The listing builds one solid part. Answer for the finished solid, in the listing's coordinates (mm). Give positions to 0.01 mm unless a question says otherwise; leave off trailing zeros. Order: outer loops, then holes, each group sorted by start corner. A loop starts at its lowest first (then second) coordinate and runs counter-clockwise, first axis right, second up.
```python
from build123d import *

# Parameters (mm, degrees)
SKETCH1_R           = 9
SKETCH1_R_2         = 2.45
SKETCH1_R_3         = 1.5
BOSS_EXTRUDE1_DEPTH = 3


with BuildPart() as part:
    # Sketch1 → Boss-Extrude1 (new body)
    with BuildSketch(Plane(origin=(0, 0, 0), x_dir=(1, 0, 0), z_dir=(0, 1, 0))):
        Circle(SKETCH1_R)
        with Locations((-5, 0.000835232)):
            Circle(SKETCH1_R_2, mode=Mode.SUBTRACT)
        with Locations((2.999131959, -5.19665349)):
            Circle(SKETCH1_R_3, mode=Mode.SUBTRACT)
        with Locations((3.000867957, 5.195651211)):
            Circle(SKETCH1_R_3, mode=Mode.SUBTRACT)
        with BuildLine():
            Line((-1.499778997, 1.323126207), (-1.500220961, -1.322625067))
            ThreePointArc((-1.500220961, -1.322625067), (1.999999972, -0.000334093), (-1.499778997, 1.323126207))
        make_face(mode=Mode.SUBTRACT)
    extrude(amount=BOSS_EXTRUDE1_DEPTH)


solid = part.part
```
1) For a pull along Z with two mould halves and no side action, classify faces 1 (the flat face through (2, 3, 2)), 2 (the cylindrical face through (2.68, 1.48, -3.73)), 3 (the cylindrical face through (-1.172, 1.479, -8.923)) as +Z half, -Z half, draft (parallel to the pull), parting line (faces both ways), or undercut.
Geometry says:
face 1: draft
face 2: undercut
face 3: parting line
2) Find section C-C (x = 2.75). Write down the section's boundary in (y, z).
Geometry says:
outline: (0, -8.57) - (3, -8.57) - (3, -6.67) - (0, -6.67) - close; (0, -3.72) - (3, -3.72) - (3, 3.72) - (0, 3.72) - close; (0, 6.68) - (3, 6.68) - (3, 8.57) - (0, 8.57) - close
3) Find section B-B (z = 5.5). Write down the section's boundary in (x, y), then the cut area to 3 significant figures.
Geometry says:
outline: (-7.12, 0) - (1.53, 0) - (1.53, 3) - (-7.12, 3) - close; (4.47, 0) - (7.12, 0) - (7.12, 3) - (4.47, 3) - close
area: 33.9 mm2
4) Find section D-D (z = -0.5). Write down the section's boundary in (x, y), then the cut area to 3 significant figures.
Geometry says:
outline: (-8.99, 0) - (-7.4, 0) - (-7.4, 3) - (-8.99, 3) - close; (-2.6, 0) - (-1.5, 0) - (-1.5, 3) - (-2.6, 3) - close; (1.94, 0) - (8.99, 0) - (8.99, 3) - (1.94, 3) - close
area: 29.2 mm2
5) Find section A-A (x = 0). Write down the section's boundary in (y, z), then the cut area to 3 significant figures.
Geometry says:
outline: (0, -9) - (3, -9) - (3, -2) - (0, -2) - close; (0, 2) - (3, 2) - (3, 9) - (0, 9) - close
area: 42.0 mm2
6) Straight lines are drawn through the part: probe 1 along X at (y, z) = (1.7, 0); probe 2 along Z at (x, y) = (1.75, 0.1); probe 3 along Z at (x, y) = (0, 0.65). For each, find the intervals that lie inside material, in ascending order.
Geometry says:
probe 1: x = -9 to -7.45, -2.55 to -1.5, 2 to 9
probe 2: z = -8.83 to -6.02, -4.37 to -0.97, 0.97 to 4.37, 6.03 to 8.83
probe 3: z = -9 to -2, 2 to 9
